Autodesk Inventor part; units mm, degrees
ref_plane "YZ Plane" through (0, 0, 0) normal (1, 0, 0) x (0, 1, 0)
ref_plane "XZ Plane" through (0, 0, 0) normal (0, 1, 0) x (-1, 0, 0)
ref_plane "XY Plane" through (0, 0, 0) normal (0, 0, 1) x (1, 0, 0)
sketch "Boceto1" plane through (0, 0, 0) normal (0, 0, 1) x (1, 0, 0)
  arc A0 (-52.25, 0) -> (52.25, 0) centre (0, 0) ccw
  line L0 (-52.25, 0) -> (-52.25, 57.25)
  line L1 (-52.25, 57.25) -> (-49.25, 57.25)
  line L2 (52.25, 57.25) -> (52.25, 0)
  arc A1 (52.25, 0) -> (-52.25, 0) centre (0, 0) ccw construction
  line L3 (0, -52.25) -> (0, 57.25) construction
  line L4 (-49.25, 57.25) -> (-49.25, 0)
  arc A2 (-49.25, 0) -> (49.25, 0) centre (0, 0) ccw
  line L5 (49.25, 0) -> (49.25, 57.25)
  line L6 (49.25, 57.25) -> (-49.25, 57.25) construction
  line L7 (49.25, 57.25) -> (49.25, 57.25)
  line L8 (-49.25, 57.25) -> (-49.25, 57.25)
  line L9 (-49.25, 57.25) -> (0, 57.25) construction
  line L10 (0, 57.25) -> (49.25, 57.25) construction
  line L11 (49.25, 57.25) -> (52.25, 57.25)
  dimension "d0" = 104.5
  dimension "d2" = 109.5
  dimension "d3" = 3
extrude "Extrusión1" add sketch "Boceto1" along normal blind 10
sketch "Boceto2" plane through (0, 0, 10) normal (0, 0, 1) x (1, 0, 0)
  line L0 (49.25, 57.25) -> (49.25, 0)
  arc A0 (-49.25, 0) -> (49.25, 0) centre (0, 0) ccw
  line L1 (-49.25, 0) -> (-49.25, 57.25)
  line L2 (-49.25, 57.25) -> (-52.25, 57.25)
  line L3 (-52.25, 57.25) -> (-52.25, 0)
  arc A1 (-52.25, 0) -> (52.25, 0) centre (0, 0) ccw
  line L4 (52.25, 0) -> (52.25, 57.25)
  line L5 (52.25, 57.25) -> (49.25, 57.25)
  line L6 (-49.25, 57.25) -> (-52.25, 57.25)
  line L7 (-52.25, 57.25) -> (-67.25, 57.25)
  line L8 (-67.25, 57.25) -> (-67.25, 54.25)
  line L9 (-67.25, 54.25) -> (-52.25, 54.25)
  line L10 (-52.25, 54.25) -> (-52.25, 57.25)
  line L11 (52.25, 57.25) -> (49.25, 57.25)
  line L12 (52.25, 57.25) -> (67.25, 57.25)
  line L13 (67.25, 57.25) -> (67.25, 54.25)
  line L14 (67.25, 54.25) -> (52.25, 54.25)
  line L15 (52.25, 54.25) -> (52.25, 57.25)
  point P0 (49.5, 57.5)
  dimension "d6" = 15
  dimension "d7" = 3
  dimension "d8" = 15
  dimension "d9" = 3
extrude "Extrusión3" add sketch "Boceto2" along normal blind 9
sketch "Boceto3" plane through (0, 0, 19) normal (0, 0, 1) x (1, 0, 0)
  line L0 (-52.25, 54.25) -> (-52.25, 0)
  line L1 (-49.25, 0) -> (-49.25, 57.25)
  line L2 (-49.25, 57.25) -> (-67.25, 57.25)
  line L3 (-67.25, 54.25) -> (-52.25, 54.25)
  line L4 (-67.25, 57.25) -> (-67.25, 54.25)
  line L5 (49.25, 57.25) -> (49.25, 0)
  line L6 (52.25, 0) -> (52.25, 54.25)
  line L7 (52.25, 54.25) -> (67.25, 54.25)
  line L8 (67.25, 54.25) -> (67.25, 57.25)
  line L9 (67.25, 57.25) -> (49.25, 57.25)
  arc A0 (-52.25, 0) -> (52.25, 0) centre (0, 0) ccw construction
  line L10 (-47.9531, -20.75) -> (47.9531, -20.75)
  arc A1 (-52.25, 0) -> (-47.9531, -20.75) centre (0, 0) ccw
  arc A2 (47.9531, -20.75) -> (52.25, 0) centre (0, 0) ccw
  arc A3 (-49.25, 0) -> (-45.9402, -17.75) centre (0, 0) ccw
  arc A4 (44.6654, -20.75) -> (45.9402, -17.75) centre (0, 0) ccw construction
  line L11 (-49.1426, -17.75) -> (-45.9402, -17.75) construction
  arc A5 (-45.9402, -17.75) -> (-44.6654, -20.75) centre (0, 0) ccw construction
  line L12 (-45.9402, -17.75) -> (45.9402, -17.75)
  arc A6 (45.9402, -17.75) -> (49.25, 0) centre (0, 0) ccw
  line L13 (45.9402, -17.75) -> (49.1426, -17.75) construction
  dimension "d14" = 78
  dimension "d15" = 3
extrude "Extrusión4" add sketch "Boceto3" along normal blind 39
sketch "Boceto4" plane through (0, 0, 19) normal (0, 0, 1) x (1, 0, 0)
  arc A0 (-47.9531, -20.75) -> (47.9531, -20.75) centre (0, 0) ccw
  line L0 (-47.9531, -20.75) -> (47.9531, -20.75)
extrude "Extrusión5" add sketch "Boceto4" along normal blind 3
sketch "Boceto5" plane through (0, 0, 58) normal (0, 0, 1) x (1, 0, 0)
  line L0 (-52.25, 54.25) -> (-52.25, 0)
  arc A0 (-52.25, 0) -> (-47.9531, -20.75) centre (0, 0) ccw
  line L1 (-47.9531, -20.75) -> (47.9531, -20.75)
  arc A1 (47.9531, -20.75) -> (52.25, 0) centre (0, 0) ccw
  line L2 (52.25, 0) -> (52.25, 54.25)
  line L3 (-52.25, 57.25) -> (-52.25, 0)
  line L4 (-52.25, 54.25) -> (-52.25, 57.25)
  line L5 (-52.25, 57.25) -> (-12.5, 57.25)
  line L6 (-12.5, 57.25) -> (-12.5, 7.25)
  line L7 (0, -5.25) -> (0, -5.25)
  line L8 (12.5, 7.25) -> (12.5, 57.25)
  line L9 (12.5, 57.25) -> (52.25, 57.25)
  line L10 (52.25, 57.25) -> (52.25, 54.25)
  arc A2 (-12.5, 7.25) -> (0, -5.25) centre (0, 7.25) ccw
  arc A3 (0, -5.25) -> (12.5, 7.25) centre (0, 7.25) ccw
  point P0 (-12.5, -5.25)
  point P1 (12.5, -5.25)
  point P2 (0, -5.25)
  dimension "d20" = 25
  dimension "d22" = 12.5
  dimension "d23" = 12.5
  dimension "d24" = 50
extrude "Extrusión6" add sketch "Boceto5" against normal blind 3
properties part number "_3DPrint"
Here's how the part is built. I have some questions about the finished solid (model axes, mm). A direction names the side the tool comes from. Round coordinates to 2 decimals unless told otherwise and drop trailing zeros. Loops run counter-clockwise (first coordinate to the right, second up) from the corner with the lowest first, then second, coordinate; pieces in that order, holes last. Notation, with made-up numbers: M 41.25,37.25 L 71.25,37.25 A8 ccw 71.25,52.25 Z; hole C 15.25,-12.75 d4. An arc over 180 degrees is marked long. Write each question's results on one line, items separated by ' | '. Start each with the question number.
(1) I want a section at A-A (y = 30). Please give me the cut outline in (x, z).
(2) I want a section at D-D (y = -42.5). Please give me the cut outline in (x, z), then the cut area to 3 significant figures.
(3) If I drill on probe 1 along X at (y, z) = (12.5, 18); probe 2 along Y at (x, z) = (57, 43); probe 3 along Z at (x, y) = (25, 23), over which ranges is the centre line in solid material (lowest first)? Write a range as from..to.
(4) I want a section at B-B (z = 45). Please give me the cut outline in (x, y).
(5) Will these pins go through, and if not, where does the flat tip stop? P1, Ø25, axis at x = -20, y = -26, coming from the -Z side; P2, Ø10, axis at y = 7.5, z = 33, coming from the -X side; P3, Ø16.5, axis at y = 33.5, z = 30.5, coming from the +X side.
(6) On a 3-axis mill with a long thin cutter (end or side, diameter ignored), from which of +Z, -Z, +X, -X, +Y, -Y can I reach the whole of each face in a straight line? I mean faces 1 (the flat face through (60, 56, 10)), 2 (the flat face through (-60, 54.25, 34)), 3 (the flat face through (-49.25, 28, 27)), 4 (the flat face through (-1, -20.75, 40)), 5 (the flat face through (12.5, 32, 57)). Say none if no direction works.
(7) I want a section at C-C (x = 16). Please give me the cut outline in (y, z), then the cut area to 3 significant figures.
Solved:
1) outline: M -52.25,0 L -49.25,0 L -49.25,55 L -12.5,55 L -12.5,58 L -52.25,58 Z; M 12.5,55 L 49.25,55 L 49.25,0 L 52.25,0 L 52.25,58 L 12.5,58 Z
2) outline: M -30.39,0 L -24.89,0 L -24.89,19 L 24.89,19 L 24.89,0 L 30.39,0 L 30.39,22 L -30.39,22 Z | area: 392 mm²
3) probe 1: x = -52.25..-49.25, 49.25..52.25 | probe 2: y = 54.25..57.25 | probe 3: z = 55..58
4) outline: M -67.25,54.25 L -52.25,54.25 L -52.25,0 A52.25 ccw -47.95,-20.75 L 47.95,-20.75 A52.25 ccw 52.25,0 L 52.25,54.25 L 67.25,54.25 L 67.25,57.25 L 49.25,57.25 L 49.25,0 A49.25 cw 45.94,-17.75 L -45.94,-17.75 A49.25 cw -49.25,0 L -49.25,57.25 L -67.25,57.25 Z
5) P1: stops at z = 19 | P2: stops at x = -52.25 | P3: stops at x = 52.25
6) face 1: -Z, +X, +Y, -Y | face 2: +Z, -Z, -X, -Y | face 3: -Z, +Y | face 4: +Z, +X, -X, -Y | face 5: +Z, -Z, +Y
7) outline: M -49.74,0 L -46.58,0 L -46.58,19 L -17.75,19 L -17.75,55 L 57.25,55 L 57.25,58 L -20.75,58 L -20.75,22 L -49.74,22 Z | area: 489 mm²
